Geometry check sheet. Reference: drawing and pictorial views, mm from the part's lowest x, y, z. Give positions to 0.01 mm unless a question says otherwise; leave off trailing zeros. Order: outer loops, then holes, each group sorted by start corner. A loop starts at its lowest first (then second) coordinate and runs counter-clockwise, first axis right, second up.
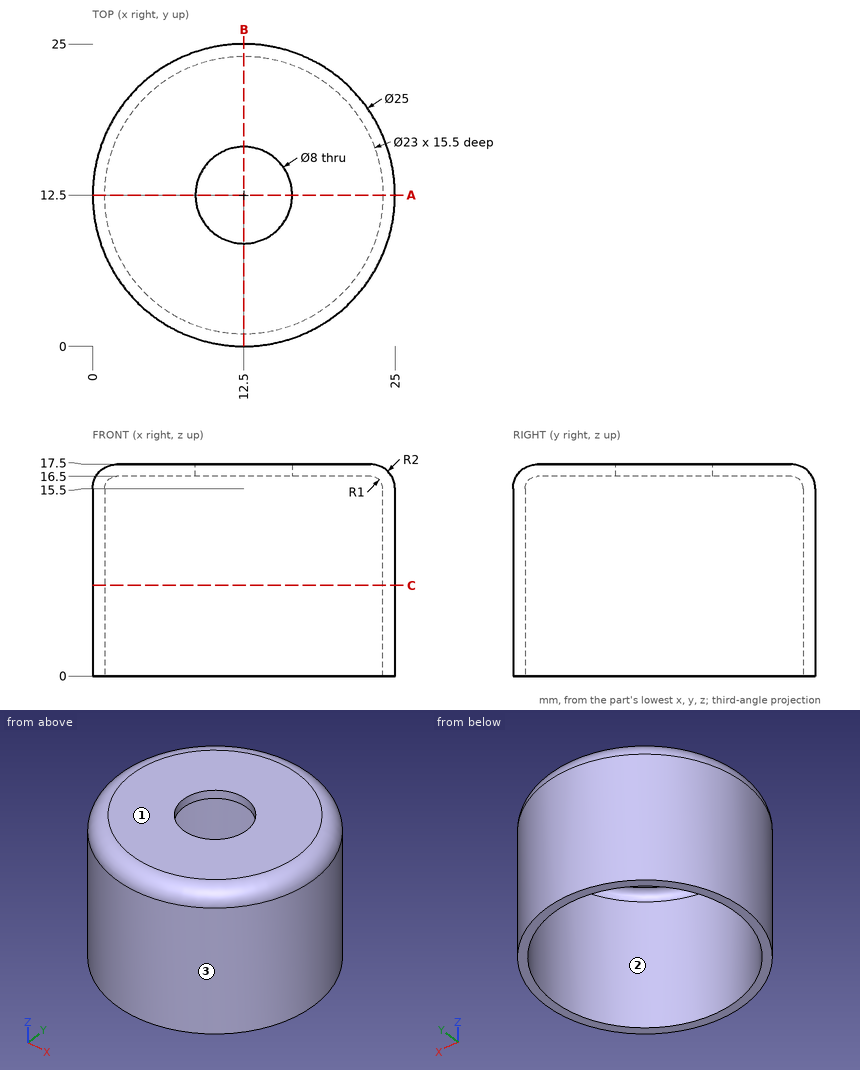
1) Draft check along Y on the marked faces 1, 2 and 3. Enter one of: +Y half, -Y half, draft (parallel to the pull), parting line (faces both ways), or undercut.
Recorded:
face 1: draft
face 2: undercut
face 3: parting line
2) Depth check by flat-ended pin: pin 1 Ø5 at (y, z) = (11, 4.5) entering from -X; pin 2 Ø5 at (y, z) = (15.5, 2.5) entering from +X; pin 3 Ø4 at (x, z) = (7, 12.5) entering from +Y; pin 4 Ø2 at (x, z) = (15.5, 13.5) entering from -Y. Enter the tip coordinate at first touch or a pass-through.
Recorded:
pin 1: stops at x = 0
pin 2: stops at x = 24.99
pin 3: stops at y = 24.5
pin 4: stops at y = 0.16
3) Material ranges on L1, parallel to Z at x = 11.75, y = 4.5; L2, parallel to Y at x = 22.5, z = 12; L3, parallel to X at y = 8.75, z = 14.5, recorded low to high.
Recorded:
L1: z = 16.5 to 17.5
L2: y = 5 to 6.82, 18.18 to 20
L3: x = 0.58 to 1.63, 23.37 to 24.42
4) Section check C-C, the plane z = 7.5. Record the cut outline in (x, y).
Recorded:
outline: circle Ø25 at (12.5, 12.5); hole circle Ø23 at (12.5, 12.5)
5) Section check A-A, the plane y = 12.5. Record the cut outline in (x, z), then the cut area to 3 significant figures.
Recorded:
outline: (0, 0) - (1, 0) - (1, 15.5) arc R1 cw to (2, 16.5) - (8.5, 16.5) - (8.5, 17.5) - (2, 17.5) arc R2 ccw to (0, 15.5) - close; (16.5, 16.5) - (23, 16.5) arc R1 cw to (24, 15.5) - (24, 0) - (25, 0) - (25, 15.5) arc R2 ccw to (23, 17.5) - (16.5, 17.5) - close
area: 48.7 mm2
